Input: part model. Units: mm. Frame: model coordinates. Face numbers are marked on the shaded views. A direction names the side the tool comes from. Give positions to 0.01 mm unless a question says otherwise; leave off trailing zeros. Loops run counter-clockwise (first coordinate to the right, second up) from the corner with the lowest first, then second, coordinate; pieces in that order, holes last.
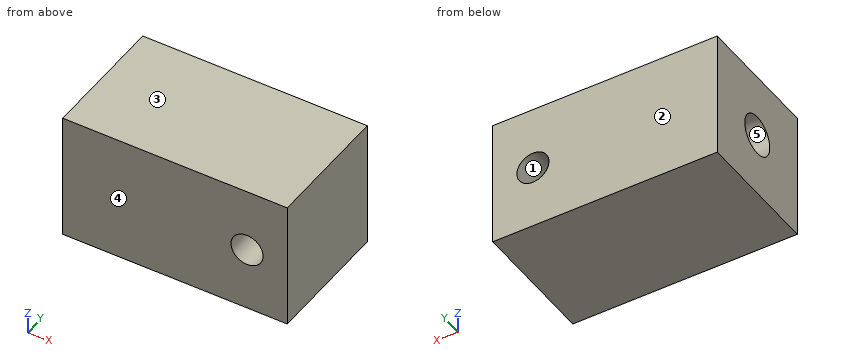
from build123d import *

# Parameters (mm, degrees)
SKETCH1_W                   = 44.45
SKETCH1_H                   = 25.4
BOSS_EXTRUDE1_DEPTH         = 25.4
SKETCH2_R                   = 3.175
CUT_EXTRUDE1_DEPTH          = 58.15
F_3_8_16_TAPPED_HOLE1_D     = 7.9375
F_3_8_16_TAPPED_HOLE1_DEPTH = 25.4
F_3_8_16_TAPPED_HOLE1_TIP   = 2.384665582


with BuildPart() as part:
    # Sketch1 → Boss-Extrude1 (new body)
    with BuildSketch(Plane(origin=(0, 0, 0), x_dir=(1, 0, 0), z_dir=(0, 1, 0))):
        with Locations((22.225, 12.7)):
            Rectangle(SKETCH1_W, SKETCH1_H)
    extrude(amount=BOSS_EXTRUDE1_DEPTH)

    # Sketch2 → Cut-Extrude1 (cut, through all)
    with BuildSketch(Plane(origin=(0, 25.4, 0), x_dir=(1, 0, 0), z_dir=(0, 1, 0))):
        with Locations(Location((36.48842715, 12.7, 0), (0, 0, 270))):
            Circle(SKETCH2_R)
    extrude(amount=-CUT_EXTRUDE1_DEPTH, mode=Mode.SUBTRACT)

    # 3/8-16 Tapped Hole1
    with Locations(Plane.ZY):
        with Locations((-12.7, 12.7)):
            Hole(F_3_8_16_TAPPED_HOLE1_D / 2, depth=F_3_8_16_TAPPED_HOLE1_DEPTH)
            with Locations((0, 0, -(F_3_8_16_TAPPED_HOLE1_DEPTH + F_3_8_16_TAPPED_HOLE1_TIP / 2))):  # 118° drill point
                Cone(0, F_3_8_16_TAPPED_HOLE1_D / 2, F_3_8_16_TAPPED_HOLE1_TIP, mode=Mode.SUBTRACT)


solid = part.part
(1) Cut plane B-B (y = 7.25). Return the cut outline in (x, z) (3 decimals), and give its area (3 significant figures).
Values follow:
outline: (0, -25.4) - (44.45, -25.4) - (44.45, 0) - (0, 0) - close; hole circle Ø6.35 at (36.488, -12.7)
area: 1,100 mm2
(2) Mould query, pull axis Z, two halves, no side actions, for the marked faces 1, 2 and 3. Classes: +Z half, -Z half, draft (parallel to the pull), parting line (faces both ways), or undercut.
Values follow:
face 1: undercut
face 2: draft
face 3: +Z half
(3) Reachability of the marked faces 4 and 5 from +Z, -Z, +X, -X, +Y, -Y: full face, straight path, thin tool, end or side. Return the list, or none.
Values follow:
face 4: +Z, -Z, +X, -X, -Y
face 5: -X
(4) Ray query, probe 1 along Y at (x, z) = (19.5, -12.7); probe 2 along X at (y, z) = (5, -11.75); probe 3 along X at (y, z) = (7, -12.7). Return the intervals inside material, ascending.
Values follow:
probe 1: y = 0 to 8.73, 16.67 to 25.4
probe 2: x = 0 to 33.46, 39.52 to 44.45
probe 3: x = 0 to 33.31, 39.66 to 44.45
(5) Cut plane A-A (x = 23). Return the cut outline in (y, z), and give its area (3 significant figures).
Values follow:
outline: (0, -25.4) - (25.4, -25.4) - (25.4, 0) - (0, 0) - close; hole circle Ø7.94 at (12.7, -12.7)
area: 596 mm2
